Here's the drawing with two shaded views (mm, measured from the low corner). I have some questions. A direction names the side the tool comes from. Coordinates: 2 decimals unless noted, no trailing zeros. Write each loop counter-clockwise with the first axis right and the second up, starting at its lowest first coordinate (ties: lowest second). Pieces come first, ordered by that corner, then holes.
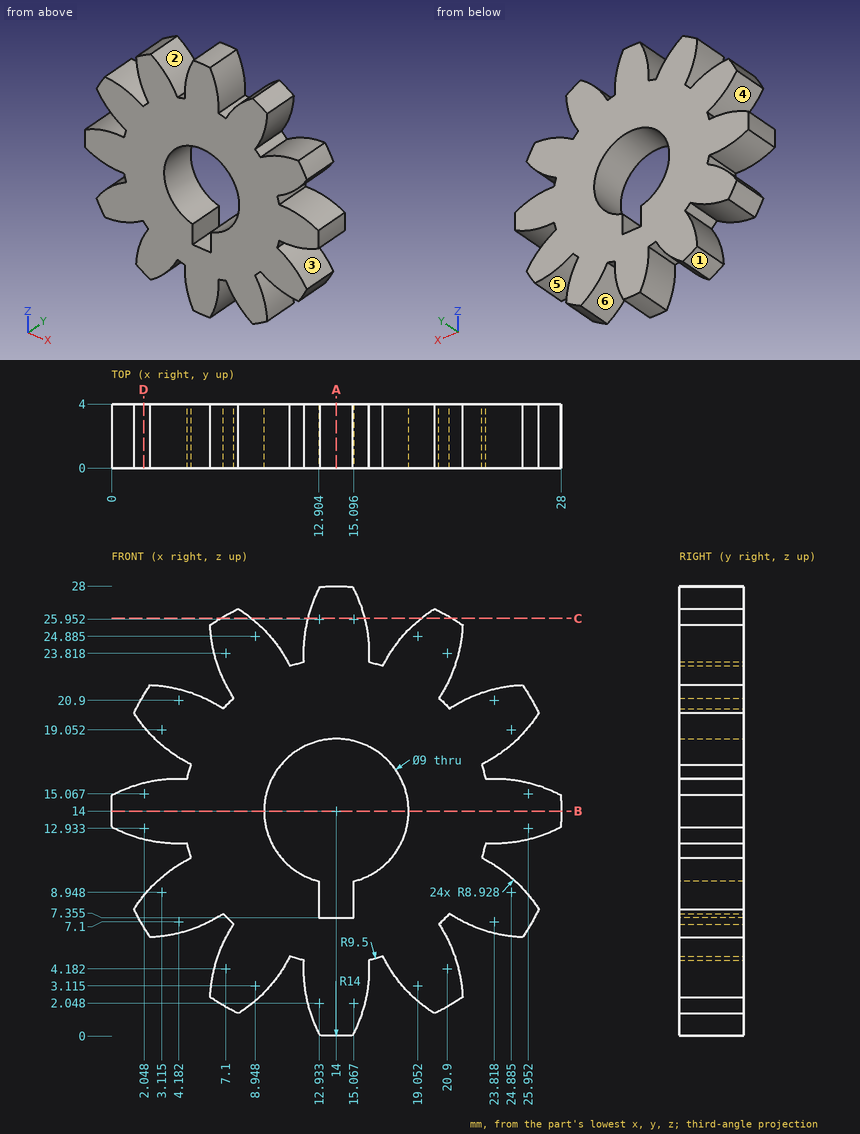
Item 1: Will these pins go through, and if not, where does the flat tip stop? pin 1 Ø1.8 at (y, z) = (1.5, 8.5) entering from +X; pin 2 Ø0.7 at (y, z) = (1.5, 8.5) entering from -X (1 decimal); pin 3 Ø1 at (y, z) = (2, 10) entering from +X (1 decimal); pin 4 Ø7 at (x, z) = (14, 14) entering from -Y (3 decimals).
Item 2: Which directions (+Z, -Z, +X, -X, +Y, -Y) give clear straight access to the entire face, cutting with the end or side of a thin tool? Please do the marked faces 4, 5 and 6.
Item 3: If I drill on line 1 along X through (y, z) = (2.05, 14); line 2 along Z through (x, y) = (20.75, 1.1) (1 decimal); line 3 along Z through (x, y) = (1.75, 2.75) (1 decimal), over which ranges is the centre line in solid material (lowest first)?
Item 4: I want a section at A-A, the plane x = 14. List the corners of the cut face in (y, z) for me (1 decimal).
Item 5: I want a section at B-B, the plane z = 14. List the corners of the cut face in (x, y) for me.
Item 6: If we mould it in two halves opening along X, with no side actions, what happens to the marked faces 1, 2 and 3? For each: released by +X, released by -X, zero draft, split by the parting line, or undercut.
Item 7: I want a section at C-C, the plane z = 26. List the corners of the cut face in (x, y) for me.
Item 8: I want a section at D-D, the plane x = 2. List the corners of the cut face in (y, z) for me.
Taken from the geometry:
1. pin 1: stops at x = 26.6
1. pin 2: stops at x = 1.6
1. pin 3: stops at x = 25.3
1. pin 4: passes through
2. face 4: -X, +Y, -Y
2. face 5: +Y, -Y
2. face 6: -Z, +Y, -Y
3. line 1: x = 0 to 9.5, 18.5 to 28
3. line 2: z = 1.7 to 6.4, 7.3 to 20.7, 21.6 to 26.3
3. line 3: z = 7.2 to 8.4, 12.3 to 15.7, 19.6 to 20.8
4. outline: (0, 0) - (4, 0) - (4, 7.4) - (0, 7.4) - close; (0, 18.5) - (4, 18.5) - (4, 28) - (0, 28) - close
5. outline: (0, 0) - (9.5, 0) - (9.5, 4) - (0, 4) - close; (18.5, 0) - (28, 0) - (28, 4) - (18.5, 4) - close
6. face 1: released by -X
6. face 2: undercut
6. face 3: released by +X
7. outline: (6.79, 0) - (8.72, 0) - (8.72, 4) - (6.79, 4) - close; (12.24, 0) - (15.76, 0) - (15.76, 4) - (12.24, 4) - close; (19.28, 0) - (21.21, 0) - (21.21, 4) - (19.28, 4) - close
8. outline: (0, 6.79) - (4, 6.79) - (4, 8.72) - (0, 8.72) - close; (0, 12.24) - (4, 12.24) - (4, 15.76) - (0, 15.76) - close; (0, 19.28) - (4, 19.28) - (4, 21.21) - (0, 21.21) - close
